Can you work these out from the model? Positions are in its coordinate system, mm. Face numbers are marked on the shaded views. A direction names the side the tool comes from. Round coordinates to 2 decimals unless told otherwise and drop trailing zeros. Write each loop counter-clockwise with the first axis right and the second up, starting at its lowest first coordinate (ties: lowest second). Pieces come first, ordered by that corner, then holes.
Q1. For the marked faces 1, 2 and 3, which set-ups out of +Z, -Z, +X, -X, +Y, -Y let a thin tool reach every point of the face, with its end or its side?
Q2. I'm going to push flat-ended pins straight in: pin 1 Ø1.6 at (x, y) = (1.5, 0) entering from -Z; pin 2 Ø3 at (x, z) = (-1.5, 4.5) entering from -Y; pin 3 Ø1.5 at (y, z) = (-5.5, -2) entering from -X; pin 4 Ø4.5 at (x, z) = (9.5, 3.5) entering from -Y. Where does each tip first touch, or does it pass through?
Q3. If we section it at B-B (x = 3.5): Please give me the cut outline in (y, z).
Q4. If we section it at D-D (z = -16.5): Please give me the cut outline in (x, y).
Q5. If we section it at C-C (z = -52): Please give me the cut outline in (x, y), plus the area to 4 significant figures.
Q6. If we section it at A-A (z = 5): Please give me the cut outline in (x, y) (3 decimals), plus the area to 3 significant figures.
Q7. Please list where these lines run through material, in increasing order: line 1 along X through (y, z) = (-3.5, 5); line 2 along X through (y, z) = (1.75, -7); line 3 along Y through (x, z) = (0.5, 0.5).
from build123d import *

# Parameters (mm, degrees)
SKETCH_1_R           = 1.525
EXTRUDE_1_DEPTH      = 10
EXTRUDE_2_DEPTH      = 2.5
EXTRUDE_2_DEPTH_BACK = 2.5
SKETCH_4_W           = 5
SKETCH_4_H           = 14
EXTRUDE_3_DEPTH      = 6.3
CUT_EXTRUDE_1_REACH  = 84.481
SKETCH_5_R           = 2.5
EXTRUDE_5_DEPTH      = 1.5


with BuildPart() as part:
    # 草图1 → 凸台-拉伸1 (new body)
    with BuildSketch(Plane.XY):
        with BuildLine():
            Line((-4.609526623, 6.301360946), (-4.609526623, 1.301360946))
            ThreePointArc((-4.609526623, 1.301360946), (-4.023740186, -0.112852616), (-2.609526623, -0.698639054))
            Line((-2.609526623, -0.698639054), (1.390473377, -0.698639054))
            Line((1.390473377, -0.698639054), (1.390473377, -7.698639054))
            Line((1.390473377, -7.698639054), (8.390473377, -7.698639054))
            Line((8.390473377, -7.698639054), (8.390473377, -0.698639054))
            Line((8.390473377, -0.698639054), (12.390473377, -0.698639054))
            ThreePointArc((12.390473377, -0.698639054), (13.804686939, -0.112852616), (14.390473377, 1.301360946))
            Line((14.390473377, 1.301360946), (14.390473377, 6.301360946))
            Line((14.390473377, 6.301360946), (-4.609526623, 6.301360946))
        make_face()
        with Locations((10.890473377, 2.801360946)):
            Circle(SKETCH_1_R, mode=Mode.SUBTRACT)
        with Locations((-1.109526623, 2.801360946)):
            Circle(SKETCH_1_R, mode=Mode.SUBTRACT)
    extrude(amount=EXTRUDE_1_DEPTH)

    # 草图3 → 凸台-拉伸2 (add, two sides: drawn at the far end of the back side and taken through both)
    with BuildSketch(Plane(origin=(4.890473377, 0, 0), x_dir=(0, 0, -1), z_dir=(1, 0, 0)).offset(-EXTRUDE_2_DEPTH_BACK)):
        Polygon((0, 6.301360946), (80, 6.301360946), (80, 1.301360946), (0, -7.698639054), align=None)
    extrude(amount=EXTRUDE_2_DEPTH + EXTRUDE_2_DEPTH_BACK)

    # 草图4 → 凸台-拉伸3 (add)
    with BuildSketch(Plane.XY.offset(10)):
        with Locations((4.890473377, -0.698639054)):
            Rectangle(SKETCH_4_W, SKETCH_4_H)
    extrude(amount=EXTRUDE_3_DEPTH)

    # 草图5 → 切除-拉伸1 (cut, up to next)
    with BuildSketch(Plane(origin=(0, 6.301360946, 0), x_dir=(1, 0, 0), z_dir=(0, 1, 0)), mode=Mode.PRIVATE) as cut_extrude_1_sk1:
        with Locations(Location((4.900882763, -5, 0), (0, 0, 270))):
            Circle(SKETCH_5_R)
    cut_extrude_1_tool1 = extrude(cut_extrude_1_sk1.sketch, amount=-CUT_EXTRUDE_1_REACH, mode=Mode.PRIVATE) & part.part
    add(cut_extrude_1_tool1.solids().sort_by_distance((4.900883, 6.301361, 5))[0], mode=Mode.SUBTRACT)

    # 草图6 → 凸台-拉伸5 (add)
    with BuildSketch(Plane(origin=(7.390473377, 0, 0), x_dir=(0, 0, -1), z_dir=(1, 0, 0))):
        Polygon((6.3, 6.301360946), (4.8, 6.301360946), (4.8, -7.158639054), (6.3, -6.989889054), align=None)
    extrude_5 = extrude(amount=EXTRUDE_5_DEPTH)

    # 镜向1: 凸台-拉伸5 across plane
    add(extrude_5.mirror(Plane(origin=(4.890473377, 0, 0), x_dir=(0, 0, 1), z_dir=(1, 0, 0))))


solid = part.part
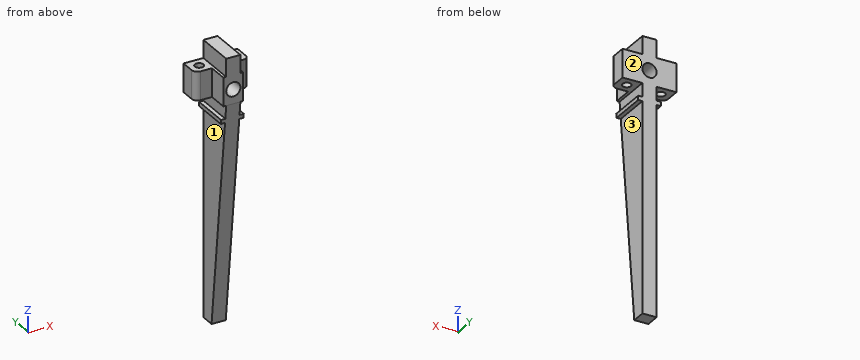
A:
1. face 1: -Z, -X, +Y, -Y
1. face 2: +Z, -Z, +X, -X, +Y
1. face 3: -Z, +X, +Y, -Y
2. pin 1: stops at z = -6.3
2. pin 2: stops at y = -0.7
2. pin 3: stops at x = 2.39
2. pin 4: stops at y = -7.7
3. outline: (-7.7, 0) - (1.3, -80) - (6.3, -80) - (6.3, 2.93) - (-7.7, 2.93) - close; (-7.7, 7.07) - (6.3, 7.07) - (6.3, 16.3) - (-7.7, 16.3) - close
4. outline: (2.39, -5.84) - (7.39, -5.84) - (7.39, 6.3) - (2.39, 6.3) - close
5. outline: (2.39, -1.85) - (7.39, -1.85) - (7.39, 6.3) - (2.39, 6.3) - close
5. area: 40.75 mm2
6. outline: (-4.61, 1.301) arc R2 ccw to (-2.61, -0.699) - (1.39, -0.699) - (1.39, -7.699) - (2.401, -7.699) - (2.401, 6.301) - (-4.61, 6.301) - close; (7.401, -7.699) - (8.39, -7.699) - (8.39, -0.699) - (12.39, -0.699) arc R2 ccw to (14.39, 1.301) - (14.39, 6.301) - (7.401, 6.301) - close; hole circle Ø3.05 at (-1.11, 2.801); hole circle Ø3.05 at (10.89, 2.801)
6. area: 95.7 mm2
7. line 1: x = 1.39 to 2.4, 7.4 to 8.39
7. line 2: x = 2.39 to 7.39
7. line 3: y = -0.7 to 6.3
